Read the model definition and answer for the solid it produces. Units are mm, in the model's axes. A direction names the side the tool comes from. Coordinates: 2 decimals unless noted, no trailing zeros. Write each loop counter-clockwise with the first axis right and the second up, starting at its lowest first coordinate (ties: lowest second). Pieces come first, ordered by that corner, then holes. Notation, with made-up numbers: M 0.25,22.5 L 26.25,22.5 A12 ccw 26.25,29.5 Z; hole C 13,73.5 d2. An arc over 180 degrees is marked long. Write item = value, one per line.
from build123d import *

# Parameters (mm, degrees)
SKETCH4_W           = 26.5
SKETCH4_H           = 26.5
BOSS_EXTRUDE2_DEPTH = 20
SHELL1_T            = -3
SKETCH6_R           = 3.9
CUT_EXTRUDE2_DEPTH  = 23.5
FILLET3_R           = 5
FILLET4_R           = 2


with BuildPart() as part:
    # Sketch4 → Boss-Extrude2 (new body)
    with BuildSketch(Plane(origin=(0, 0, 0), x_dir=(0, 1, 0), z_dir=(0, 0, 1))):
        Rectangle(SKETCH4_W, SKETCH4_H)
    extrude(amount=BOSS_EXTRUDE2_DEPTH)

    # Shell1
    shell1_openings = [part.faces().sort_by_distance(p)[0] for p in [
        (0, 0, 20),
        (0, 13.25, 10),
        (0, -13.25, 10),
    ]]
    offset(amount=SHELL1_T, openings=shell1_openings, kind=Kind.INTERSECTION)

    # Sketch6 → Cut-Extrude2 (cut)
    with BuildSketch(Plane.YZ.offset(13.25)):
        with Locations((-7.8, 10)):
            Circle(SKETCH6_R)
        with Locations((7.8, 10)):
            Circle(SKETCH6_R)
    extrude(amount=-CUT_EXTRUDE2_DEPTH, mode=Mode.SUBTRACT)

    # Fillet3
    fillet3_edges = [part.edges().sort_by_distance(p)[0] for p in [
        (-13.25, 0, 0),
        (13.25, 0, 0),
    ]]
    fillet(fillet3_edges, radius=FILLET3_R)

    # Fillet4
    fillet4_edges = [part.edges().sort_by_distance(p)[0] for p in [
        (10.25, 0, 3),
        (-10.25, 0, 3),
    ]]
    fillet(fillet4_edges, radius=FILLET4_R)


solid = part.part
Item 1: Find section B-B (y = -4.5). Determine the outline of the cut face in (x, z), and give its area (3 significant figures).
Worked answers:
outline = M -13.25,5 A5 ccw -8.25,0 L 8.25,0 A5 ccw 13.25,5 L 13.25,7.92 L 10.25,7.92 L 10.25,5 A2 cw 8.25,3 L -8.25,3 A2 cw -10.25,5 L -10.25,20 L -13.25,20 Z; M 10.25,12.08 L 13.25,12.08 L 13.25,20 L 10.25,20 Z
area = 160 mm²
Item 2: Find section C-C (z = 17.25). Determine the outline of the cut face in (x, y).
Worked answers:
outline = M -13.25,-13.25 L -10.25,-13.25 L -10.25,13.25 L -13.25,13.25 Z; M 10.25,-13.25 L 13.25,-13.25 L 13.25,13.25 L 10.25,13.25 Z
Item 3: Find section D-D (y = 2.5). Determine the outline of the cut face in (x, z), and give its area (3 significant figures).
Worked answers:
outline = M -13.25,5 A5 ccw -8.25,0 L 8.25,0 A5 ccw 13.25,5 L 13.25,20 L 10.25,20 L 10.25,5 A2 cw 8.25,3 L -8.25,3 A2 cw -10.25,5 L -10.25,20 L -13.25,20 Z
area = 172 mm²
Item 4: Which of the six approach directions +Z, -Z, +X, -X, +Y, -Y give full straight-line access (tool end or side, diameter ignored) to faces 1 (the face through (11.771, -5.703, 13.288)), 2 (the face through (11.82, 0.19, 1.5)), 3 (the face through (-9.68, 0.19, 3.6))?
Worked answers:
face_1 = +X
face_2 = -Z, +X, +Y, -Y
face_3 = +Z, +Y, -Y
Item 5: Consider line 1 along X through (y, z) = (0.25, 8); line 2 along X through (y, z) = (5.5, 8.5); line 3 along Z through (x, y) = (0, 9.5). Determine where each line is inside the solid, lowest interval first. Write a range as from..to.
Worked answers:
line_1 = -13.25..-10.25, 10.25..13.25
line_2 = -13.25..-10.25
line_3 = 0..3
Item 6: Flat-ended cylindrical pins translate along their axes: pin 1 (4 mm diameter, centred on x = -4, y = -8, fed in from +Z); pin 2 (2 mm diameter, centred on x = -8.5, z = 5, fed in from -Y); pin 3 (10 mm diameter, centred on x = 6.5, z = 11.5, fed in from +Y). Find the tip coordinate at first contact, or state that the pin passes through.
Worked answers:
pin_1 = 3
pin_2 = through
pin_3 = 13.25
Item 7: For a pull along X with two mould halves and no side action, classify faces 4 (the face through (-11.75, 0.19, 1.43)), 5 (the face through (0.1, -13.25, 2.5)), 6 (the face through (9.65, 0.19, 3.57)) as released by +X, released by -X, zero draft, split by the parting line, or undercut.
Worked answers:
face_4 = released by -X
face_5 = zero draft
face_6 = undercut
Item 8: Find section A-A (z = 10). Determine the outline of the cut face in (x, y), and give its area (3 significant figures).
Worked answers:
outline = M -13.25,-13.25 L -10.25,-13.25 L -10.25,13.25 L -13.25,13.25 Z; M 10.25,-13.25 L 13.25,-13.25 L 13.25,-11.7 L 10.25,-11.7 Z; M 10.25,-3.9 L 13.25,-3.9 L 13.25,3.9 L 10.25,3.9 Z; M 10.25,11.7 L 13.25,11.7 L 13.25,13.25 L 10.25,13.25 Z
area = 112 mm²
